```python
from build123d import *

# Parameters (mm, degrees)
ESBO_O1_R                = 14.32
RESSALTO_EXTRUS_O1_DEPTH = 7.9
ESBO_O2_R                = 6.255
CORTE_EXTRUS_O1_DEPTH    = 7.9
ESBO_O3_R                = 12.41
ESBO_O3_R_2              = 8.6
CORTE_EXTRUS_O2_DEPTH    = 0.24


with BuildPart() as part:
    # Esboço1 → Ressalto-extrusão1 (new body)
    with BuildSketch(Plane(origin=(0, 0, 0), x_dir=(1, 0, 0), z_dir=(0, 1, 0))):
        with Locations(Location((-2.489539578, 0, 0), (0, 0, 270))):
            Circle(ESBO_O1_R)
    extrude(amount=RESSALTO_EXTRUS_O1_DEPTH)

    # Esboço2 → Corte-extrusão1 (cut)
    with BuildSketch(Plane(origin=(0, 7.9, 0), x_dir=(1, 0, 0), z_dir=(0, 1, 0))):
        with Locations(Location((-2.489539578, 0, 0), (0, 0, 270))):
            Circle(ESBO_O2_R)
    extrude(amount=-CORTE_EXTRUS_O1_DEPTH, mode=Mode.SUBTRACT)

    # Esboço3 → Corte-extrusão2 (cut)
    with BuildSketch(Plane(origin=(0, 7.9, 0), x_dir=(1, 0, 0), z_dir=(0, 1, 0))):
        with Locations(Location((-2.489539578, 0, 0), (0, 0, 270))):
            Circle(ESBO_O3_R)
        with Locations(Location((-2.489539578, 0, 0), (0, 0, 270))):
            Circle(ESBO_O3_R_2, mode=Mode.SUBTRACT)
    corte_extrus_o2 = extrude(amount=-CORTE_EXTRUS_O2_DEPTH, mode=Mode.SUBTRACT)

    # Espelhar1: Corte-extrusão2 across plane
    add(corte_extrus_o2.mirror(Plane.ZX.offset(3.95)), mode=Mode.SUBTRACT)


solid = part.part
```
Read the model definition and answer for the solid it produces. Units are mm, in the model's axes. A direction names the side the tool comes from. Coordinates: 2 decimals unless noted, no trailing zeros. Loops run counter-clockwise (first coordinate to the right, second up) from the corner with the lowest first, then second, coordinate; pieces in that order, holes last. Notation, with made-up numbers: (73.25, 3) - (98.25, 3) arc R33 ccw to (98.25, 31) - close; hole circle Ø1 at (57, 71.5). An arc over 180 degrees is marked (long way). Answer in a Markdown table with one row per item.
1. Determine the mould class of faces 1 (the face through (11.71, 3.89, -1.86)), 2 (the face through (-6.3, 4.01, -4.96)), 3 (the face through (4, 7.9, -11)) for opening direction Z: +Z half, -Z half, draft (parallel to the pull), parting line (faces both ways), or undercut.
Conclusion:
| item | result |
|---|---|
| face 1 | parting line |
| face 2 | undercut |
| face 3 | draft |
2. Given pin 1 (1.5 mm diameter, centred on x = -11.5, z = -5.5, fed in from +Y); pin 2 (3 mm diameter, centred on y = 6.5, z = -7, fed in from +X); pin 3 (3 mm diameter, centred on y = 2, z = -3.5, fed in from +X), each flat-ended and moving along its own axis, determine where each tip first touches the part or whether it passes through.
Conclusion:
| item | result |
|---|---|
| pin 1 | stops at y = 7.66 |
| pin 2 | stops at x = 10.73 |
| pin 3 | stops at x = 11.69 |
3. Find section B-B, the plane x = -7.75. Write down the section's boundary in (y, z), then the cut area to 3 significant figures.
Conclusion:
| item | result |
|---|---|
| outline | (0, -13.32) - (7.9, -13.32) - (7.9, -11.24) - (7.66, -11.24) - (7.66, -6.8) - (7.9, -6.8) - (7.9, -3.38) - (0, -3.38) - (0, -6.8) - (0.24, -6.8) - (0.24, -11.24) - (0, -11.24) - close; (0, 3.38) - (7.9, 3.38) - (7.9, 6.8) - (7.66, 6.8) - (7.66, 11.24) - (7.9, 11.24) - (7.9, 13.32) - (0, 13.32) - (0, 11.24) - (0.24, 11.24) - (0.24, 6.8) - (0, 6.8) - close |
| area | 153 mm² |
4. Straight lines are drawn through the part: line 1 (X direction, y = 7.85, z = 0); line 2 (X direction, y = 5.75, z = 0); line 3 (Z direction, x = -2.5, y = 6) (3 decimals). For each, find the intervals that lie inside material, in ascending order.
Conclusion:
| item | result |
|---|---|
| line 1 | x = -16.81 to -14.9, -11.09 to -8.74, 3.77 to 6.11, 9.92 to 11.83 |
| line 2 | x = -16.81 to -8.74, 3.77 to 11.83 |
| line 3 | z = -14.32 to -6.255, 6.255 to 14.32 |
5. Find section C-C, the plane y = 5. Write down the section's boundary in (x, z) (3 decimals), then the cut area to 3 significant figures.
Conclusion:
| item | result |
|---|---|
| outline | circle Ø28.64 at (-2.49, 0); hole circle Ø12.51 at (-2.49, 0) |
| area | 521 mm² |
6. Find section A-A, the plane z = 0. Write down the section's boundary in (x, y).
Conclusion:
| item | result |
|---|---|
| outline | (-16.81, 0) - (-14.9, 0) - (-14.9, 0.24) - (-11.09, 0.24) - (-11.09, 0) - (-8.74, 0) - (-8.74, 7.9) - (-11.09, 7.9) - (-11.09, 7.66) - (-14.9, 7.66) - (-14.9, 7.9) - (-16.81, 7.9) - close; (3.77, 0) - (6.11, 0) - (6.11, 0.24) - (9.92, 0.24) - (9.92, 0) - (11.83, 0) - (11.83, 7.9) - (9.92, 7.9) - (9.92, 7.66) - (6.11, 7.66) - (6.11, 7.9) - (3.77, 7.9) - close |
7. Which of the six approach directions +Z, -Z, +X, -X, +Y, -Y give full straight-line access (tool end or side, diameter ignored) to faces 4 (the face through (-11, 0.24, -3)), 5 (the face through (-11, 7.66, -3)), 6 (the face through (4, 0, -11))?
Conclusion:
| item | result |
|---|---|
| face 4 | -Y |
| face 5 | +Y |
| face 6 | +Z, -Z, +X, -X, -Y |
8. Find section D-D, the plane z = -9. Write down the section's boundary in (x, y).
Conclusion:
| item | result |
|---|---|
| outline | (-13.63, 0) - (-11.03, 0) - (-11.03, 0.24) - (6.05, 0.24) - (6.05, 0) - (8.65, 0) - (8.65, 7.9) - (6.05, 7.9) - (6.05, 7.66) - (-11.03, 7.66) - (-11.03, 7.9) - (-13.63, 7.9) - close |
